Can you work these out from the model? Positions are in its coordinate system, mm. A direction names the side the tool comes from. Give positions to 0.01 mm unless a question says otherwise; leave off trailing zeros. Order: outer loops, then holes, each group sorted by start corner. A loop starts at its lowest first (then second) coordinate and runs counter-clockwise, first axis right, second up. Notation, with made-up numbers: (43, 15.5) - (78, 15.5) arc R27 cw to (78, 37.5) - close; hole circle Ø9 at (83, 11.25). An arc over 180 degrees is marked (long way). One line per question, with ' | ' between items.
```python
from build123d import *

# Parameters (mm, degrees)
SKETCH1_R           = 5
SKETCH1_R_2         = 3
BOSS_EXTRUDE1_DEPTH = 5
BOSS_EXTRUDE2_DEPTH = 3
SKETCH3_R           = 1.5
CUT_EXTRUDE1_DEPTH  = 3
SKETCH4_R           = 3
CUT_EXTRUDE2_DEPTH  = 3
CUT_EXTRUDE3_DEPTH  = 10


with BuildPart() as part:
    # Sketch1 → Boss-Extrude1 (new body)
    with BuildSketch(Plane.XY):
        Circle(SKETCH1_R)
        Circle(SKETCH1_R_2, mode=Mode.SUBTRACT)
    extrude(amount=BOSS_EXTRUDE1_DEPTH)

    # Sketch2 → Boss-Extrude2 (add)
    with BuildSketch(Plane.XY.offset(5)):
        with BuildLine():
            Line((-30, 4), (0, 7))
            ThreePointArc((0, 7), (7, 0), (0, -7))
            Line((0, -7), (-30, -4))
            ThreePointArc((-30, -4), (-34, 0), (-30, 4))
        make_face()
    extrude(amount=BOSS_EXTRUDE2_DEPTH)

    # Sketch3 → Cut-Extrude1 (cut)
    with BuildSketch(Plane(origin=(0, 0, 5), x_dir=(-1, 0, 0), z_dir=(0, 0, -1))):
        with Locations((25, 0)):
            Circle(SKETCH3_R)
    extrude(amount=-CUT_EXTRUDE1_DEPTH, mode=Mode.SUBTRACT)

    # Sketch4 → Cut-Extrude2 (cut)
    with BuildSketch(Plane(origin=(0, 0, 5), x_dir=(-1, 0, 0), z_dir=(0, 0, -1))):
        Circle(SKETCH4_R)
    extrude(amount=-CUT_EXTRUDE2_DEPTH, mode=Mode.SUBTRACT)

    # Sketch5 → Cut-Extrude3 (cut)
    with BuildSketch(Plane(origin=(0, 0, 5), x_dir=(-1, 0, 0), z_dir=(0, 0, -1))):
        with BuildLine():
            Line((27.128027058, 4.287197294), (27.128027058, 0))
            Line((27.128027058, 0), (27.128027058, -4.287197294))
            Line((27.128027058, -4.287197294), (30, -4))
            ThreePointArc((30, -4), (34, 0), (30, 4))
            Line((30, 4), (27.128027058, 4.287197294))
        make_face()
    extrude(amount=-CUT_EXTRUDE3_DEPTH, mode=Mode.SUBTRACT)


solid = part.part
```
(1) If I drill on line 1 (Y direction, x = 0, z = 1.9); line 2 (X direction, y = 1.25, z = 7.25); line 3 (Z direction, x = -8.5, y = 3.75), over which ranges is the centre line in solid material (lowest first)?
Answer below:
line 1: -5 to -3, 3 to 5 | line 2: -27.13 to -25.83, -24.17 to -2.73, 2.73 to 6.89 | line 3: 5 to 8
(2) Will these pins go through, and if not, where does the flat tip stop? pin 1 (5 mm diameter, centred on x = -25, y = 0, fed in from -Z); pin 2 (2 mm diameter, centred on y = -2.5, z = 2.5, fed in from -X).
Answer below:
pin 1: z = 5 | pin 2: x = -4.77
(3) Imagine slicing it at D-D (y = -3.5). List the corners of the cut face in (x, z) for me.
Answer below:
outline: (-27.13, 5) - (-3.57, 5) - (-3.57, 0) - (3.57, 0) - (3.57, 5) - (6.06, 5) - (6.06, 8) - (-27.13, 8) - close
(4) Imagine slicing it at B-B (x = -25). List the corners of the cut face in (y, z) for me.
Answer below:
outline: (-4.5, 5) - (-1.5, 5) - (-1.5, 8) - (-4.5, 8) - close; (1.5, 5) - (4.5, 5) - (4.5, 8) - (1.5, 8) - close
(5) Imagine slicing it at A-A (y = 0). List the corners of the cut face in (x, z) for me.
Answer below:
outline: (-27.13, 5) - (-26.5, 5) - (-26.5, 8) - (-27.13, 8) - close; (-23.5, 5) - (-5, 5) - (-5, 0) - (-3, 0) - (-3, 8) - (-23.5, 8) - close; (3, 0) - (5, 0) - (5, 5) - (7, 5) - (7, 8) - (3, 8) - close
(6) If we mould it in two halves opening along X, with no side actions, what happens to faces 3 (the face through (-23.5, 0.07, 6.48)), 4 (the face through (7, 0, 6)), 5 (the face through (-10, 0, 8)), 6 (the face through (-27.128, 0, 6))? For each: released by +X, released by -X, zero draft, split by the parting line, or undercut.
Answer below:
face 3: undercut | face 4: released by +X | face 5: zero draft | face 6: released by -X
(7) On a 3-axis mill with a long thin cutter (end or side, diameter ignored), from which of +Z, -Z, +X, -X, +Y, -Y can I reach the whole of each face in a straight line? I mean faces 1 (the face through (-1.08, -4.88, 2.46)), 2 (the face through (-0.1, -3.3, 0)). Say none if no direction works.
Answer below:
face 1: -Z | face 2: -Z, +X, -X, +Y, -Y
(8) Imagine slicing it at C-C (z = 3.75). List the corners of the cut face in (x, y) for me, and give its area (3 significant figures).
Answer below:
outline: circle Ø10 at (0, 0); hole circle Ø6 at (0, 0) | area: 50.3 mm^2
